Work out the finished part from the listing and answer in its coordinate system (mm). Face numbers are marked on the shaded views. A direction names the side the tool comes from. Coordinates: 2 decimals unless noted, no trailing zeros. Loops run counter-clockwise (first coordinate to the right, second up) from the corner with the lowest first, then second, coordinate; pieces in that order, holes last. Notation, with made-up numbers: (-35.75, 66) -> (-6.75, 66) arc R25 ccw to (-6.75, 81) -> close; hole circle Ø8 at (-26, 39.5). An arc over 180 degrees is marked (long way). Use a Markdown table: item, result.
from build123d import *

# Parameters (mm, degrees)
BOSS_EXTRUDE1_DEPTH = 50
SKETCH3_R           = 3.05
CUT_EXTRUDE1_DEPTH  = 7.5
SKETCH4_R           = 5.25
CUT_EXTRUDE2_DEPTH  = 50
SKETCH5_W           = 148.528027858
SKETCH5_H           = 40
CUT_EXTRUDE3_DEPTH  = 40


with BuildPart() as part:
    # Sketch2 → Boss-Extrude1 (new body)
    with BuildSketch(Plane(origin=(0, 0, 0), x_dir=(1, 0, 0), z_dir=(0, 1, 0))):
        with BuildLine():
            Line((-75, 30), (75, 30))
            Line((75, 30), (75, -30))
            Line((75, -30), (-55.05, -30))
            Line((-55.05, -30), (-55.05, -5))
            ThreePointArc((-55.05, -5), (-75, 14.95), (-94.95, -5))
            Line((-94.95, -5), (-110, -5))
            ThreePointArc((-110, -5), (-99.748737342, 19.748737342), (-75, 30))
        make_face()
    extrude(amount=BOSS_EXTRUDE1_DEPTH)

    # Sketch3 → Cut-Extrude1 (cut)
    with BuildSketch(Plane.XY.offset(5)):
        with Locations((-102.475, 40)):
            Circle(SKETCH3_R)
        with Locations((-102.475, 10)):
            Circle(SKETCH3_R)
    extrude(amount=-CUT_EXTRUDE1_DEPTH, mode=Mode.SUBTRACT)

    # Sketch4 → Cut-Extrude2 (cut)
    with BuildSketch(Plane.XY.offset(-2.5)):
        with Locations((-102.475, 40)):
            Circle(SKETCH4_R)
        with Locations((-102.475, 10)):
            Circle(SKETCH4_R)
    extrude(amount=-CUT_EXTRUDE2_DEPTH, mode=Mode.SUBTRACT)

    # Sketch5 → Cut-Extrude3 (cut)
    with BuildSketch(Plane(origin=(0, 50, 0), x_dir=(1, 0, 0), z_dir=(0, 1, 0))):
        with Locations((29.214013929, 0)):
            Rectangle(SKETCH5_W, SKETCH5_H)
    extrude(amount=-CUT_EXTRUDE3_DEPTH, mode=Mode.SUBTRACT)


solid = part.part
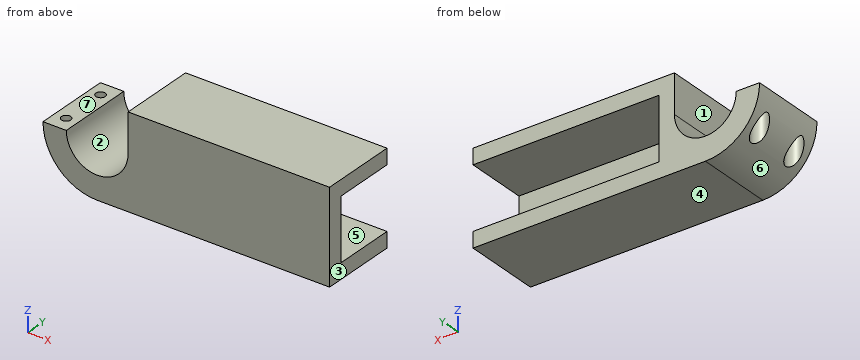
Q1. Section D-D on z = 15.5 is taken. Determine the outline of the cut face in (x, y).
Solved:
| item | result |
|---|---|
| outline | (-55.05, 0) -> (75, 0) -> (75, 10) -> (-45.05, 10) -> (-45.05, 50) -> (-55.05, 50) -> close |
Q2. Section A-A on z = 3 is taken. State how many separate pieces and enclosed holes the cut face has, and give its area (3 significant figures).
Solved:
| item | result |
|---|---|
| separate pieces | 2 |
| enclosed holes | 2 |
| area | 2,400 mm² |
Q3. Given pin 1 Ø6 at (y, z) = (12, 0) entering from -X; pin 2 Ø20 at (y, z) = (24, -7.5) entering from +X; pin 3 Ø3 at (x, y) = (-103.5, 38) entering from -Z; pin 4 Ø3.5 at (x, y) = (-102.475, 40) entering from -Z, each flat-ended and moving along its own axis, determine where each tip first touches the part or whether it passes through.
Solved:
| item | result |
|---|---|
| pin 1 | x = -109.94 |
| pin 2 | x = -45.05 |
| pin 3 | z = -2.5 |
| pin 4 | through |
Q4. Consider line 1 (Z direction, x = -33, y = 25.5); line 2 (X direction, y = 6, z = 4); line 3 (X direction, y = 3, z = 20.5). Determine where each line is inside the solid, lowest interval first. Write a range as [from, to].
Solved:
| item | result |
|---|---|
| line 1 | [-30, -20], [20, 30] |
| line 2 | [-109.99, -94.92], [-55.08, 75] |
| line 3 | [-55.05, 75] |
Q5. Section C-C on x = 22 is taken. Determine the outline of the cut face in (y, z), and give its area (3 significant figures).
Solved:
| item | result |
|---|---|
| outline | (0, -30) -> (50, -30) -> (50, -20) -> (10, -20) -> (10, 20) -> (50, 20) -> (50, 30) -> (0, 30) -> close |
| area | 1,400 mm² |
Q6. Determine the mould class of the marked faces 1, 2, 3 and 4 for opening direction X: pulls with the +X half, pulls with the -X half, needs draft (parallel to the pull), parting line crosses it, or undercut.
Solved:
| item | result |
|---|---|
| face 1 | pulls with the -X half |
| face 2 | undercut |
| face 3 | pulls with the +X half |
| face 4 | needs draft |
Q7. For the marked faces 5, 6 and 7, determine the directions among +Z, -Z, +X, -X, +Y, -Y from which every point of the face is accessible in a straight line to the end or side of a thin tool.
Solved:
| item | result |
|---|---|
| face 5 | +X, +Y |
| face 6 | -Z, -X, +Y, -Y |
| face 7 | +Z, -X, +Y, -Y |
Q8. Section B-B on y = 3 is taken. Determine the outline of the cut face in (x, z).
Solved:
| item | result |
|---|---|
| outline | (-110, 5) arc R35 ccw to (-75, -30) -> (75, -30) -> (75, 30) -> (-55.05, 30) -> (-55.05, 5) arc R19.95 cw to (-94.95, 5) -> close |
